The listing builds one solid part. Answer for the finished solid, in the listing's coordinates (mm). Face numbers are marked on the shaded views. A direction names the side the tool comes from. Round coordinates to 2 decimals unless told otherwise and drop trailing zeros. Write each loop counter-clockwise with the first axis right and the second up, starting at its lowest first coordinate (ties: lowest second). Pieces come first, ordered by that corner, then holes. Notation, with made-up numbers: (78.25, -19) - (84.25, -19) arc R21 ccw to (84.25, -1) - close; hole circle Ø5 at (45.25, 48). An arc over 180 degrees is marked (long way). Return JSON: item names as keys, results as strings. Group by question number.
(1) Section B-B, the plane x = -240.5 is taken. Write down the section's boundary in (y, z), then the cut area to 3 significant figures.
(2) Section A-A, the plane z = 43 is taken. Write down the section's boundary in (x, y).
(3) Determine the mould class of the marked faces 1, 2 and 3 for opening direction X: +X half, -X half, draft (parallel to the pull), parting line (faces both ways), or undercut.
(4) Section C-C, the plane y = 94.5 is taken. Write down the section's boundary in (x, z).
(5) Each of these flat-tipped pins is pushed along its axis until it touches: pin 1 (6.5 mm diameter, centred on y = -0.5, z = 4.5, fed in from +X); pin 2 (6 mm diameter, centred on x = 150.5, y = -127.5, fed in from -Z); pin 3 (12 mm diameter, centred on y = -85.5, z = 37, fed in from -X). Where does it stop, or does it pass through?
(6) Find the intervals of material crossed by line 1 along Y through (x, z) = (74, 37); line 2 along X through (y, z) = (-28, 94); line 3 along Y through (x, z) = (-114, 123.5), in increasing order. Write a range as [from, to].
(7) Which of the six approach directions +Z, -Z, +X, -X, +Y, -Y give full straight-line access (tool end or side, diameter ignored) to the marked faces 4, 5, 6 and 7?
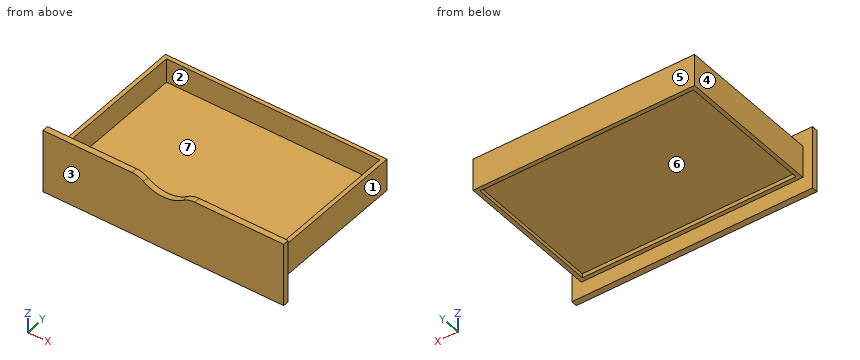
```python
from build123d import *

# Parameters (mm, degrees)
F0_W     = 673.1
F0_H     = 12.7
F1_DEPTH = 101.6
F3_E11_W = 673.1
F3_E11_H = 431.8
F4_DEPTH = 12.7
F5_W     = 698.5
F5_H     = 101.6
F6_DEPTH = 19.05


with BuildPart() as f1:
    # F0 (on Top) → F1 (new body)
    with BuildSketch(Plane.XY):
        Polygon((336.55, 215.9), (349.25, 228.6), (-349.25, 228.6), (-336.55, 215.9), align=None)
        Polygon((349.25, -228.6), (349.25, 228.6), (336.55, 215.9), (336.55, -215.9), (336.55, -228.6), align=None)
        Polygon((-336.55, 215.9), (-349.25, 228.6), (-349.25, -228.6), (-336.55, -228.6), (-336.55, -215.9), align=None)
        with Locations((0, -222.25)):
            Rectangle(F0_W, F0_H)
    extrude(amount=F1_DEPTH)

    # F3_E11 (on explicit) → F4 (join)
    with BuildSketch(Plane(origin=(336.55, 215.9, 12.7), x_dir=(-1, 0, 0), z_dir=(0, 0, 1))):
        with Locations((336.55, 215.9)):
            Rectangle(F3_E11_W, F3_E11_H)
    extrude(amount=F4_DEPTH)

    # F5 (on face) → F6 (join)
    with BuildSketch(Plane.XZ.offset(228.6)):
        with BuildLine():
            Line((-379.476, -49.276), (379.476, -49.276))
            Line((379.476, -49.276), (379.476, 150.876))
            Line((379.476, 150.876), (99.0458770515, 150.876))
            ThreePointArc((99.0458770515, 150.876), (79.7868016321, 147.884991183), (62.3420274532, 139.1937327241))
            ThreePointArc((62.3420274532, 139.1937327241), (0, 119.3512302291), (-62.3420274532, 139.1937327241))
            ThreePointArc((-62.3420274532, 139.1937327241), (-79.7868016321, 147.884991183), (-99.0458770515, 150.876))
            Line((-99.0458770515, 150.876), (-379.476, 150.876))
            Line((-379.476, 150.876), (-379.476, -49.276))
        make_face()
        with Locations((0, 50.8)):
            Rectangle(F5_W, F5_H, mode=Mode.SUBTRACT)
        with Locations((0, 50.8)):
            Rectangle(F5_W, F5_H)
    extrude(amount=F6_DEPTH)


solid = f1.part
```
Working result:
{
 "1": {"outline": "(-247.65, -49.28) - (-228.6, -49.28) - (-228.6, 0) - (-215.9, 0) - (-215.9, 12.7) - (215.9, 12.7) - (215.9, 0) - (228.6, 0) - (228.6, 101.6) - (215.9, 101.6) - (215.9, 25.4) - (-215.9, 25.4) - (-215.9, 101.6) - (-228.6, 101.6) - (-228.6, 150.88) - (-247.65, 150.88) - close", "area": "11,900 mm^2"},
 "2": {"outline": "(-379.48, -247.65) - (379.48, -247.65) - (379.48, -228.6) - (349.25, -228.6) - (349.25, 228.6) - (-349.25, 228.6) - (-349.25, -228.6) - (-379.48, -228.6) - close; hole (-336.55, -215.9) - (336.55, -215.9) - (336.55, 215.9) - (-336.55, 215.9) - close"},
 "3": {"face 1": "+X half", "face 2": "undercut", "face 3": "draft"},
 "4": {"outline": "(-349.25, 0) - (-336.55, 0) - (-336.55, 12.7) - (336.55, 12.7) - (336.55, 0) - (349.25, 0) - (349.25, 101.6) - (336.55, 101.6) - (336.55, 25.4) - (-336.55, 25.4) - (-336.55, 101.6) - (-349.25, 101.6) - close"},
 "5": {"pin 1": "stops at x = 349.25", "pin 2": "stops at z = 12.7", "pin 3": "stops at x = -349.25"},
 "6": {"line 1": "y = [-247.65, -215.9], [215.9, 228.6]", "line 2": "x = [-349.25, -336.55], [336.55, 349.25]", "line 3": "y = [-247.65, -228.6]"},
 "7": {"face 4": "+Z, -Z, -X, +Y", "face 5": "+Z, -Z, +X, -X, +Y", "face 6": "-Z", "face 7": "+Z"}
}
